Verification items for the finished model (mm, model axes). Round coordinates to 2 decimals unless told otherwise and drop trailing zeros. Write each loop counter-clockwise with the first axis right and the second up, starting at its lowest first coordinate (ties: lowest second). Pieces come first, ordered by that corner, then holes. Notation, with made-up numbers: M -13.5,-27 L 42.5,-27 A25 cw 42.5,-11 Z; hole C 41.5,64.5 d7. An arc over 180 degrees is marked long. One line per item, written item: value. Start each with the question number.
Item 1: Section check B-B, the plane x = 12.5. Record the cut outline in (y, z).
Item 2: Section check C-C, the plane z = 44. Record the cut outline in (x, y), then the cut area to 3 significant figures.
Item 3: Section check D-D, the plane y = 12. Record the cut outline in (x, z), then the cut area to 3 significant figures.
Item 4: Thickness scan on probe 1 along Y at (x, z) = (72, -25.5); probe 2 along Z at (x, y) = (30.5, 8); probe 3 along X at (y, z) = (6.5, 23). Record the ranges inside material, lowest first. Write a range as from..to.
Item 5: Gauge pin test, flat ends, axial feed: pin 1 (2 mm diameter, centred on x = 62.5, y = 26, fed in from +Z); pin 2 (8 mm diameter, centred on y = 12, z = -29, fed in from -X); pin 3 (3 mm diameter, centred on x = 72.898, z = 0, fed in from -Y). Record the tip position at first contact, or that the pin passes through.
Item 6: Section check A-A, the plane y = 28.5. Record the cut outline in (x, z), then the cut area to 3 significant figures.
from build123d import *

# Parameters (mm, degrees)
F0_W      = 93.019191
F0_H      = 32.043829
F1_DEPTH  = 64.77
F2_R      = 15.330256
F3_W      = 34.98908
F3_H      = 2.32445
F4_DEPTH  = 72.898
F4_FACE_W = 72.898
F4_FACE_H = 34.98908


with BuildPart() as f1:
    # F0 (on Top) → F1 (new body)
    with BuildSketch(Plane.XY):
        with Locations((-10.116236, -0.464286)):
            Rectangle(F0_W, F0_H)
    extrude(amount=F1_DEPTH)

    # F2
    f2_edges = [f1.edges().sort_by_distance(p)[0] for p in [
        (-10.116236, -16.486201, 64.77),
    ]]
    fillet(f2_edges, radius=F2_R)

    # F3 (on Right) → F4 (join)
    with BuildSketch(Plane.YZ):
        with Locations((32.786973, -1.162225)):
            Rectangle(F3_W, F3_H)
    extrude(amount=F4_DEPTH)

    # F4_face (on face) → F5 (revolve)
    with BuildSketch(Plane(origin=(36.449, 32.786973, -2.32445), x_dir=(1, 0, 0), z_dir=(0, 0, -1))):
        Rectangle(F4_FACE_W, F4_FACE_H)
    revolve(axis=Axis((72.898, 32.786973, 0), (0, -1, 0)))


solid = f1.part
Response values:
1. outline: M -16.49,0 L 15.29,0 L 15.29,-40.89 L 50.28,-40.89 L 50.28,40.89 L 15.56,40.89 L 15.56,64.77 L -1.16,64.77 A15.33 ccw -16.49,49.44 Z
2. outline: M -56.63,-16.49 L 36.39,-16.49 L 36.39,15.29 L 131.07,15.29 L 131.07,50.28 L 14.73,50.28 L 14.73,15.56 L -56.63,15.56 Z
2. area: 7,050 mm2
3. outline: M -56.63,0 L 36.39,0 L 36.39,64.77 L -56.63,64.77 Z
3. area: 6,020 mm2
4. probe 1: y = 15.29..50.28
4. probe 2: z = 0..64.77
4. probe 3: x = -56.63..36.39
5. pin 1: stops at z = 72.33
5. pin 2: stops at x = 5.04
5. pin 3: stops at y = 15.29
6. outline: C 72.9,0 d145.87; hole M 70.57,0 L 72.9,0 L 72.9,-2.32 A2.32 ccw long Z
6. area: 16,700 mm2
